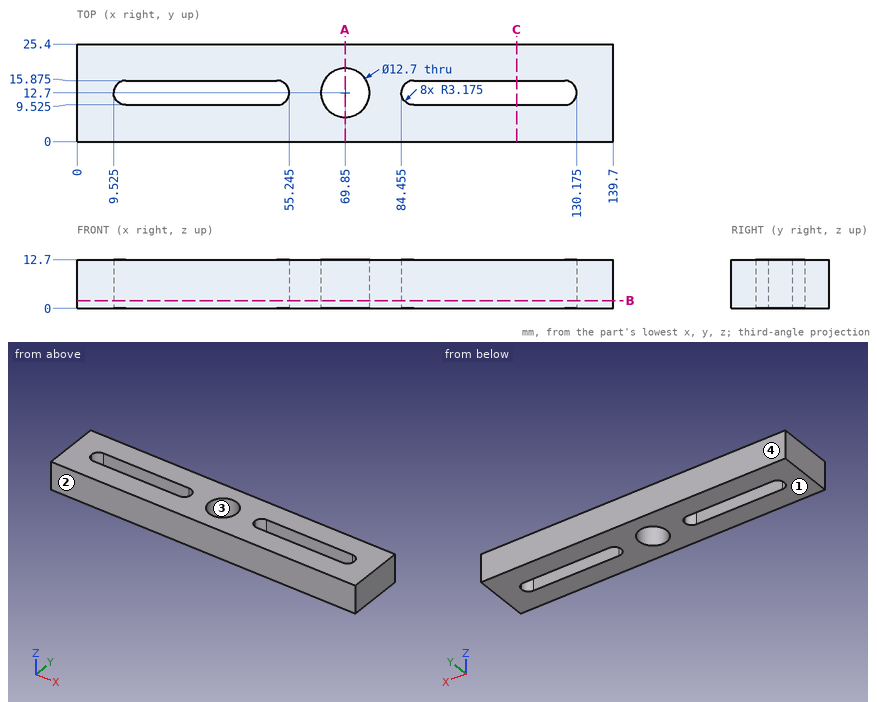
Geometry: see drawing. Coordinates: mm, zero at the bounding-box minimum. Give positions to 0.01 mm unless a question says otherwise; leave off trailing zeros. Loops run counter-clockwise (first coordinate to the right, second up) from the corner with the lowest first, then second, coordinate; pieces in that order, holes last. Notation, with made-up numbers: (68.25, 2) - (111.25, 2) arc R9 cw to (111.25, 8) - close; hole circle Ø9 at (83.5, 42). An arc over 180 degrees is marked (long way). Use CSV: the item, a comma, the result in double quotes. Start each with the question number.
Item 1: Section C-C on x = 114.5. Return loops of the section in (y, z) (3 decimals), then the cut area to 3 significant figures.
Item 2: Section B-B on z = 2. State how many separate pieces and enclosed holes the cut face has, then the cut area to 3 significant figures.
Item 3: Line query: line 1 (X direction, y = 13, z = 4.5); line 2 (Y direction, x = 114.5, z = 8.75) (3 decimals); line 3 (Y direction, x = 69.85, z = 8). Output: solid intervals per line, ascending.
Item 4: Section A-A on x = 69.85. Return loops of the section in (y, z).
Item 5: Mould query, pull axis Y, two halves, no side actions, for the marked faces 1, 2, 3 and 4. Classes: pulls with the +Y half, pulls with the -Y half, needs draft (parallel to the pull), parting line crosses it, or undercut.
Item 6: Contact query for a flat-ended pin moving along its axis: P1, Ø1, axis at x = 22.5, y = 14, coming from the -Z side. Output: stop coordinate, or through.
Ans:
1,outline,"(0, 0) - (9.525, 0) - (9.525, 12.7) - (0, 12.7) - close; (15.875, 0) - (25.4, 0) - (25.4, 12.7) - (15.875, 12.7) - close"
1,area,"242 mm2"
2,separate pieces,"1"
2,enclosed holes,"3"
2,area,"2,860 mm2"
3,line 1,"x = 0 to 9.54, 55.23 to 63.51, 76.19 to 84.47, 130.16 to 139.7"
3,line 2,"y = 0 to 9.525, 15.875 to 25.4"
3,line 3,"y = 0 to 6.35, 19.05 to 25.4"
4,outline,"(0, 0) - (6.35, 0) - (6.35, 12.7) - (0, 12.7) - close; (19.05, 0) - (25.4, 0) - (25.4, 12.7) - (19.05, 12.7) - close"
5,face 1,"needs draft"
5,face 2,"pulls with the -Y half"
5,face 3,"undercut"
5,face 4,"pulls with the +Y half"
6,P1,"passes through"
